from build123d import *

# Parameters (mm, degrees)
BOSS_EXTRUDE1_DEPTH     = 11.5
BOSS_EXTRUDE2_DEPTH     = 90
SKETCH3_W               = 56
SKETCH3_H               = 56
BOSS_EXTRUDE3_DEPTH     = 10
SKETCH4_W               = 10
SKETCH4_H               = 0.6
SKETCH5_W               = 10
SKETCH5_H               = 0.6
SKETCH6_W               = 10
SKETCH6_H               = 0.6
SKETCH7_W               = 10
SKETCH7_H               = 0.6
HOLE1_D                 = 5.6
HOLE1_DEPTH             = 5
HOLE2_D                 = 5.6
HOLE2_DEPTH             = 5
CUT_EXTRUDE9_DEPTH      = 110.759965379
CUT_EXTRUDE9_DEPTH_BACK = 5
FILLET3_R               = 2
FILLET4_R               = 3
SKETCH17_R              = 4
BOSS_EXTRUDE4_DEPTH     = 12


with BuildPart() as part:
    # Sketch1 → Boss-Extrude1 (new body)
    with BuildSketch(Plane(origin=(0, 0, 0), x_dir=(-1, 0, 0), z_dir=(0, 0, -1))):
        Polygon((-23, 28), (-28, 23), (-28, -23), (-23, -28), (23, -28), (28, -23), (28, 23), (23, 28), align=None)
    extrude(amount=-BOSS_EXTRUDE1_DEPTH)

    # Sketch2 → Boss-Extrude2 (add)
    with BuildSketch(Plane.XY.offset(11.5)):
        Polygon((23, 28), (-23, 28), (-28, 23), (-28, -23), (-23, -28), (23, -28), (28, -23), (28, 23), align=None)
    extrude(amount=BOSS_EXTRUDE2_DEPTH)

    # Sketch3 → Boss-Extrude3 (add)
    with BuildSketch(Plane.XY.offset(101.5)):
        Rectangle(SKETCH3_W, SKETCH3_H)
    extrude(amount=BOSS_EXTRUDE3_DEPTH)

    # Sketch4 → Revolve1 (revolve)
    with BuildSketch(Plane.XY.offset(3.65)):
        with Locations((-26, 0.95)):
            Rectangle(SKETCH4_W, SKETCH4_H)
    revolve(axis=Axis((-31, 0.65, 3.65), (1, 0, 0)))

    # Sketch5 → Revolve2 (revolve)
    with BuildSketch(Plane.XY.offset(3.65)):
        with Locations((-26, -0.35)):
            Rectangle(SKETCH5_W, SKETCH5_H)
    revolve(axis=Axis((-31, -0.65, 3.65), (1, 0, 0)))

    # Sketch6 → Revolve3 (revolve)
    with BuildSketch(Plane.XY.offset(4.95)):
        with Locations((-26, -0.35)):
            Rectangle(SKETCH6_W, SKETCH6_H)
    revolve(axis=Axis((-31, -0.65, 4.95), (1, 0, 0)))

    # Sketch7 → Revolve4 (revolve)
    with BuildSketch(Plane.XY.offset(4.95)):
        with Locations((-26, 0.95)):
            Rectangle(SKETCH7_W, SKETCH7_H)
    revolve(axis=Axis((-31, 0.65, 4.95), (1, 0, 0)))

    # Sketch8 → Revolve5 (revolve)
    with BuildSketch(Plane.XZ, mode=Mode.PRIVATE) as revolve5_sk:
        Polygon((4, 133.5), (0, 133.5), (0, 111.5), (19, 111.5), (19, 113.5), (4, 113.5), align=None)
    revolve(revolve5_sk.sketch.rotate(Axis((0, 0, 133.5), (0, 0, -1)), 180), axis=Axis((0, 0, 133.5), (0, 0, -1)))

    # Hole1
    with Locations(Plane.XY.offset(111.5)):
        with Locations((-23.55, 23.55)):
            hole1 = Hole(HOLE1_D / 2, depth=HOLE1_DEPTH)

    # Hole2
    with Locations(Plane.XY.offset(111.5)):
        with Locations((-23.55, -23.55), (-23.55, 23.55)):
            hole2 = Hole(HOLE2_D / 2, depth=HOLE2_DEPTH)

    # Mirror2: Hole1, Hole2 across plane
    add(hole1.mirror(Plane(origin=(0, 0, 0), x_dir=(0, 0, 1), z_dir=(1, 0, 0))), mode=Mode.SUBTRACT)
    add(hole2.mirror(Plane(origin=(0, 0, 0), x_dir=(0, 0, 1), z_dir=(1, 0, 0))), mode=Mode.SUBTRACT)

    # Sketch34 → Cut-Extrude9 (cut, two sides: drawn at the far end of the back side and taken through both)
    with BuildSketch(Plane(origin=(0, 0, 101.5), x_dir=(-1, 0, 0), z_dir=(0, 0, -1)).offset(-CUT_EXTRUDE9_DEPTH_BACK)):
        with BuildLine():
            Line((18.55, 23.55), (18.55, 34.67124832))
            Line((18.55, 34.67124832), (31.974713938, 34.67124832))
            Line((31.974713938, 34.67124832), (31.974713938, 18.55))
            Line((31.974713938, 18.55), (23.55, 18.55))
            ThreePointArc((23.55, 18.55), (20.014466094, 20.014466094), (18.55, 23.55))
        make_face()
        with BuildLine():
            Line((23.55, -18.55), (31.974713938, -18.55))
            Line((31.974713938, -18.55), (31.974713938, -34.67124832))
            Line((31.974713938, -34.67124832), (18.55, -34.67124832))
            Line((18.55, -34.67124832), (18.55, -23.55))
            ThreePointArc((18.55, -23.55), (20.014466094, -20.014466094), (23.55, -18.55))
        make_face()
        with BuildLine():
            Line((-18.55, -23.55), (-18.55, -34.67124832))
            Line((-18.55, -34.67124832), (-31.974713938, -34.67124832))
            Line((-31.974713938, -34.67124832), (-31.974713938, -18.55))
            Line((-31.974713938, -18.55), (-23.55, -18.55))
            ThreePointArc((-23.55, -18.55), (-20.014466094, -20.014466094), (-18.55, -23.55))
        make_face()
        with BuildLine():
            Line((-23.55, 18.55), (-31.974713938, 18.55))
            Line((-31.974713938, 18.55), (-31.974713938, 34.67124832))
            Line((-31.974713938, 34.67124832), (-18.55, 34.67124832))
            Line((-18.55, 34.67124832), (-18.55, 23.55))
            ThreePointArc((-18.55, 23.55), (-20.014466094, 20.014466094), (-23.55, 18.55))
        make_face()
    extrude(amount=CUT_EXTRUDE9_DEPTH + CUT_EXTRUDE9_DEPTH_BACK, mode=Mode.SUBTRACT)

    # Fillet3
    fillet3_edges = [part.edges().sort_by_distance(p)[0] for p in [
        (18.55, 28, 53.25),
        (28, 18.55, 53.25),
        (28, -18.55, 53.25),
        (18.55, -28, 53.25),
        (-18.55, -28, 53.25),
        (-28, -18.55, 53.25),
        (-28, 18.55, 53.25),
        (-18.55, 28, 53.25),
    ]]
    fillet(fillet3_edges, radius=FILLET3_R)

    # Fillet4
    fillet4_edges = [part.edges().sort_by_distance(p)[0] for p in [
        (28, -28, 109),
        (28, 28, 109),
        (-28, 28, 109),
        (-28, -28, 109),
    ]]
    fillet(fillet4_edges, radius=FILLET4_R)

    # Sketch17 → Boss-Extrude4 (add)
    with BuildSketch(Plane(origin=(0, 0, 0), x_dir=(-1, 0, 0), z_dir=(0, 0, -1))):
        Circle(SKETCH17_R)
    extrude(amount=BOSS_EXTRUDE4_DEPTH)


solid = part.part
Here's how the part is built. I have some questions about the finished solid (model axes, mm). A direction names the side the tool comes from. Give positions to 0.01 mm unless a question says otherwise; leave off trailing zeros. Loops run counter-clockwise (first coordinate to the right, second up) from the corner with the lowest first, then second, coordinate; pieces in that order, holes last. Notation, with made-up numbers: (-20.75, 17.25) -> (-8.75, 17.25) arc R27 ccw to (-8.75, 42.25) -> close; hole circle Ø5 at (8.25, -33.75). An arc over 180 degrees is marked (long way). Answer as a JSON object with one key per item and string values. Group by question number.
Item 1: Will these pins go through, and if not, where does the flat tip stop? pin 1 (1.5 mm diameter, centred on x = 21.5, z = 19, fed in from +Y); pin 2 (6.5 mm diameter, centred on x = -23.55, y = -23.55, fed in from -Z); pin 3 (2 mm diameter, centred on y = 0.5, z = 29, fed in from -X); pin 4 (3.5 mm diameter, centred on x = -23, y = -23.5, fed in from -Z).
Item 2: On a 3-axis mill with a long thin cutter (end or side, diameter ignored), from which of +Z, -Z, +X, -X, +Y, -Y can I reach the whole of each face in a straight line? I mean faces 5 (the flat face through (-24.9, 26.2, 106.5)), 6 (the flat face through (22, -21, 106.5)), 7 (the flat face through (20.9, 24.9, 106.5)), 8 (the cylindrical face through (4.119, -18.548, 112.514)). Say none if no direction works.
Item 3: Imagine slicing it at C-C on y = 6.5. Write out the boundary of the cut face in (x, z).
Item 4: Imagine slicing it at D-D on x = -12.5. Write out the boundary of the cut face in (y, z).
Item 5: Imagine slicing it at B-B on x = 2.5. Write out the boundary of the cut face in (y, z), then the cut area to 3 significant figures.
Item 6: Imagine slicing it at A-A on z = 88.5. Write out the boundary of the cut face in (x, y), then the cut area to 3 significant figures.
Item 7: I need wall thicknesses on L1, parallel to Y at x = 23.55, z = 107.8; L2, parallel to X at y = -23, z = 108; L3, parallel to Z at x = -13.5, y = 16.5. Which ranges of each line are inside material? Lowest first, please.
Item 8: Thinking about a two-plate mould opening in Y: for faces 1 (the flat face through (0, 28, 55)), 2 (the cylindrical face through (21.328, -25.254, 108.965)), 3 (the cylindrical face through (21.486, 25.442, 108.965)), 4 (the flat face through (0.3, 4.5, 113.5)), which applies, pulls with the +Y half, pulls with the -Y half, needs draft (parallel to the pull), parting line crosses it, or undercut?
Answer list:
{
 "1": {"pin 1": "stops at y = 19.41", "pin 2": "stops at z = 106.5", "pin 3": "stops at x = -28", "pin 4": "passes through"},
 "2": {"face 5": "-Z, -X, +Y", "face 6": "-Z, +X, -Y", "face 7": "-Z, +X, +Y", "face 8": "+Z"},
 "3": {"outline": "(-28, 0) -> (28, 0) -> (28, 111.5) -> (17.85, 111.5) -> (17.85, 113.5) -> (-17.85, 113.5) -> (-17.85, 111.5) -> (-28, 111.5) -> close"},
 "4": {"outline": "(-28, 0) -> (28, 0) -> (28, 111.5) -> (14.31, 111.5) -> (14.31, 113.5) -> (-14.31, 113.5) -> (-14.31, 111.5) -> (-28, 111.5) -> close"},
 "5": {"outline": "(-28, 0) -> (-3.12, 0) -> (-3.12, -12) -> (3.12, -12) -> (3.12, 0) -> (28, 0) -> (28, 111.5) -> (18.83, 111.5) -> (18.83, 113.5) -> (3.12, 113.5) -> (3.12, 133.5) -> (-3.12, 133.5) -> (-3.12, 113.5) -> (-18.83, 113.5) -> (-18.83, 111.5) -> (-28, 111.5) -> close", "area": "6,520 mm2"},
 "6": {"outline": "(-28, -16.55) arc R2 ccw to (-26, -18.55) -> (-23.55, -18.55) arc R5 cw to (-18.55, -23.55) -> (-18.55, -26) arc R2 ccw to (-16.55, -28) -> (16.55, -28) arc R2 ccw to (18.55, -26) -> (18.55, -23.55) arc R5 cw to (23.55, -18.55) -> (26, -18.55) arc R2 ccw to (28, -16.55) -> (28, 16.55) arc R2 ccw to (26, 18.55) -> (23.55, 18.55) arc R5 cw to (18.55, 23.55) -> (18.55, 26) arc R2 ccw to (16.55, 28) -> (-16.55, 28) arc R2 ccw to (-18.55, 26) -> (-18.55, 23.55) arc R5 cw to (-23.55, 18.55) -> (-26, 18.55) arc R2 ccw to (-28, 16.55) -> close", "area": "2,790 mm2"},
 "7": {"L1": "y = -28 to -26.35, -20.75 to 20.75, 26.35 to 28", "L2": "x = -28 to -26.3, -20.8 to 20.8, 26.3 to 28", "L3": "z = 0 to 111.5"},
 "8": {"face 1": "pulls with the +Y half", "face 2": "undercut", "face 3": "undercut", "face 4": "needs draft"}
}
